Read the model definition and answer for the solid it produces. Units are mm, in the model's axes. Face numbers are marked on the shaded views. A direction names the side the tool comes from. Give positions to 0.01 mm unless a question says otherwise; leave off trailing zeros. Order: outer loops, then holes, each group sorted by start corner. A loop starts at its lowest first (then second) coordinate and runs counter-clockwise, first axis right, second up. Notation, with made-up numbers: (0.25, 39.5) - (13.25, 39.5) arc R31 ccw to (13.25, 70.5) - close; hole circle Ø2 at (49, 88.25). An arc over 180 degrees is marked (long way). Return JSON: item names as keys, results as strings.
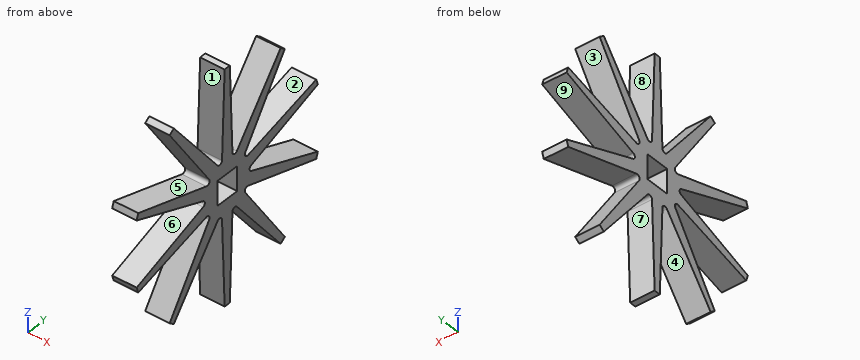
Autodesk Inventor part; units mm, degrees
ref_plane "YZ Plane" through (0, 0, 0) normal (1, 0, 0) x (0, 1, 0)
ref_plane "XZ Plane" through (0, 0, 0) normal (0, 1, 0) x (-1, 0, 0)
ref_plane "XY Plane" through (0, 0, 0) normal (0, 0, 1) x (1, 0, 0)
sketch "Sketch1" plane through (0, 0, 0) normal (1, 0, 0) x (0, 1, 0)
  circle A0 centre (0, 0) radius 60.325
  line L0 (-6.35, 6.35) -> (6.35, 6.35)
  line L1 (6.35, 6.35) -> (6.35, -6.35)
  line L2 (6.35, -6.35) -> (-6.35, -6.35)
  line L3 (-6.35, -6.35) -> (-6.35, 6.35)
  line L4 (-6.35, 6.35) -> (0, 0) construction
  line L5 (0, 0) -> (6.35, 6.35) construction
  line L6 (-6.35, -6.35) -> (0, 0) construction
  line L7 (0, 0) -> (6.35, -6.35) construction
  dimension "d0" = 120.65
  dimension "d1" = 12.7
extrude "Extrusion1" add sketch "Sketch1" along normal blind 12.7
sketch "Sketch2" plane through (12.7, 0, 0) normal (1, 0, 0) x (0, 0, -1)
  circle A0 centre (0, 0) radius 60.325
  line L0 (0, 0) -> (0, 60.325) construction
  line L1 (0, 60.325) -> (-17.056, 57.8636) construction
  line L2 (0, 60.325) -> (17.056, 57.8636) construction
  line L3 (17.056, 57.8636) -> (0, 0) construction
  line L4 (0, 0) -> (-17.056, 57.8636) construction
  arc A1 (17.056, 57.8636) -> (-17.056, 57.8636) centre (0, 0) ccw construction
  line L5 (-17.056, 57.8636) -> (-1.4908, 15.3294)
  line L6 (1.4908, 15.3294) -> (17.056, 57.8636)
  arc A2 (-1.4908, 15.3294) -> (1.4908, 15.3294) centre (0, 15.875) ccw
  dimension "d4" = 32.847
  dimension "d11" = 1.5875
  dimension "d12" = 44.45
extrude "Extrusion3" cut sketch "Sketch2" against normal through all contours L6 A2 L5 A0 picked at (-9.0544, 44.2998)
pattern_circular "Circular Pattern2" count 10 over 360 about axis through (0, 0, 0) along (1, 0, 0) of "Extrusion3"
properties part number "IntakeRoller" material "Silicone"
Q1. Determine the mould class of the marked faces 1, 2, 3 and 4 for opening direction Z: released by +Z, released by -Z, zero draft, split by the parting line, or undercut.
Values:
{"face 1": "released by +Z", "face 2": "undercut", "face 3": "undercut", "face 4": "released by -Z"}
Q2. Given pin 1 (4 mm diameter, centred on x = 9.5, y = -1, fed in from -Z) (3 decimals); pin 2 (6 mm diameter, centred on x = 5, y = 31.5, fed in from -Z), each flat-ended and moving along its own axis, determine where each tip first touches the part or whether it passes through.
Values:
{"pin 1": "stops at z = -60.325", "pin 2": "stops at z = -49.76"}
Q3. A cutting plane is placed at C-C (z = -18.5). Write down the section's boundary in (x, y).
Values:
{"outline": "(0, -57.42) - (12.7, -57.42) - (12.7, -50.83) - (0, -50.83) - close; (0, -17.09) - (12.7, -17.09) - (12.7, -9.59) - (0, -9.59) - close; (0, -3.19) - (12.7, -3.19) - (12.7, 3.19) - (0, 3.19) - close; (0, 9.59) - (12.7, 9.59) - (12.7, 17.09) - (0, 17.09) - close; (0, 50.83) - (12.7, 50.83) - (12.7, 57.42) - (0, 57.42) - close"}
Q4. A cutting plane is placed at A-A (z = 24). Write down the section's boundary in (x, y), and give its area (3 significant figures).
Values:
{"outline": "(0, -20.79) - (12.7, -20.79) - (12.7, -13.9) - (0, -13.9) - close; (0, -2.99) - (12.7, -2.99) - (12.7, 2.99) - (0, 2.99) - close; (0, 13.9) - (12.7, 13.9) - (12.7, 20.79) - (0, 20.79) - close", "area": "251 mm²"}
Q5. Consider L1, parallel to Y at x = 4, z = -34; L2, parallel to Y at x = 8.25, z = -37; L3, parallel to Z at x = 3.5, y = -34. Determine where each line is inside the solid, lowest interval first.
Values:
{"L1": "y = -27.51 to -21.74, -2.62 to 2.62, 21.74 to 27.51", "L2": "y = -29.52 to -24.1, -2.51 to 2.51, 24.1 to 29.52", "L3": "z = -49.63 to -43.66, -13.71 to -8.32, 8.32 to 13.71, 43.66 to 49.63"}
Q6. A cutting plane is placed at B-B (y = 32.5). Write down the section's boundary in (x, z), and give its area (3 significant figures).
Values:
{"outline": "(0, -47.72) - (12.7, -47.72) - (12.7, -41.43) - (0, -41.43) - close; (0, -13.28) - (12.7, -13.28) - (12.7, -7.77) - (0, -7.77) - close; (0, 7.77) - (12.7, 7.77) - (12.7, 13.28) - (0, 13.28) - close; (0, 41.43) - (12.7, 41.43) - (12.7, 47.72) - (0, 47.72) - close", "area": "300 mm²"}
Q7. A cutting plane is placed at D-D (y = -22). Write down the section's boundary in (x, z).
Values:
{"outline": "(0, -34.33) - (12.7, -34.33) - (12.7, -25.8) - (0, -25.8) - close; (0, -10.29) - (12.7, -10.29) - (12.7, -3.93) - (0, -3.93) - close; (0, 3.93) - (12.7, 3.93) - (12.7, 10.29) - (0, 10.29) - close; (0, 25.8) - (12.7, 25.8) - (12.7, 34.33) - (0, 34.33) - close"}
Q8. For the marked faces 5, 6, 7, 8 and 9, determine the directions among +Z, -Z, +X, -X, +Y, -Y from which every point of the face is accessible in a straight line to the end or side of a thin tool.
Values:
{"face 5": "+X, -X", "face 6": "+X, -X, -Y", "face 7": "-Z, +X, -X", "face 8": "+Z, +X, -X", "face 9": "+X, -X, +Y"}
